Work out the finished part from the listing and answer in its coordinate system (mm). Face numbers are marked on the shaded views. A direction names the side the tool comes from. Coordinates: 2 decimals unless noted, no trailing zeros. Write each loop counter-clockwise with the first axis right and the second up, starting at its lowest first coordinate (ties: lowest second). Pieces come first, ordered by that corner, then holes. Notation, with made-up numbers: (28.5, 66) - (73.5, 66) arc R22 cw to (73.5, 77) - close; hole circle Ø1 at (11, 13). An arc over 180 degrees is marked (long way). Use a Markdown table: item, result. Add a question column.
(1) Find the intervals of material crossed by line 1 (X direction, y = 2.5, z = -1); line 2 (X direction, y = 5.5, z = -2); line 3 (X direction, y = 1.9, z = 6.75), in increasing order. Write a range as from..to.
(2) The part is cut by section B-B, the plane x = 20. Give the vertices of the cut face in (y, z).
(3) The part is cut by section C-C, the plane y = 1. Give the vertices of the cut face in (x, z).
(4) The part is cut by section A-A, the plane z = 0. Give the vertices of the cut face in (x, y), then the cut area to 4 significant figures.
(5) Given pin 1 Ø5.5 at (x, z) = (-20, 0) entering from -Y; pin 2 Ø2 at (x, y) = (5, 0.5) entering from +Z; pin 3 Ø2.5 at (x, y) = (4, 2) entering from -Z; pin 4 Ø3 at (x, y) = (-15.5, 1) entering from +Z, each flat-ended and moving along its own axis, determine where each tip first touches the part or whether it passes through.
(6) For a pull along X with two mould halves and no side action, classify the marked faces 4 and 5 as released by +X, released by -X, zero draft, split by the parting line, or undercut.
(7) A tool of negligible diameter and unlimited length cuts with its end or side. For the marked faces 1, 2 and 3, from which of +Z, -Z, +X, -X, +Y, -Y can it reach the whole face along a straight path? Write none if from no direction.
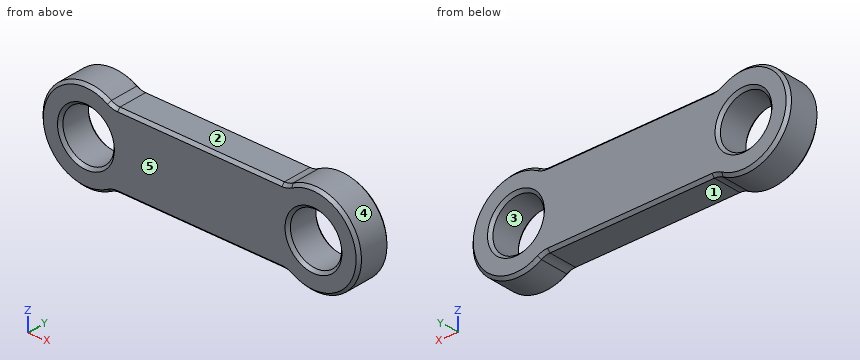
from build123d import *

# Parameters (mm, degrees)
SKETCH_1_R      = 4.5
EXTRUDE_1_DEPTH = 6
FILLET_1_R      = 3
CHAMFER_1_SIZE  = 0.5


with BuildPart() as part:
    # 草图1 → 凸台-拉伸1 (new body)
    with BuildSketch(Plane(origin=(0, 0, 0), x_dir=(1, 0, 0), z_dir=(0, 1, 0))):
        with BuildLine():
            Line((-15.336310473, 6.5), (15.336310473, 6.5))
            ThreePointArc((15.336310473, 6.5), (28, 0), (15.336310473, -6.5))
            Line((15.336310473, -6.5), (-15.336310473, -6.5))
            ThreePointArc((-15.336310473, -6.5), (-28, 0), (-15.336310473, 6.5))
        make_face()
        with Locations(Location((-20, 0, 0), (0, 0, 270))):
            Circle(SKETCH_1_R, mode=Mode.SUBTRACT)
        with Locations(Location((20, 0, 0), (0, 0, 270))):
            Circle(SKETCH_1_R, mode=Mode.SUBTRACT)
    extrude(amount=EXTRUDE_1_DEPTH)

    # 圆角1
    fillet_1_edges = [part.edges().sort_by_distance(p)[0] for p in [
        (-15.336310473, 3, -6.5),
        (15.336310473, 3, -6.5),
        (15.336310473, 3, 6.5),
        (-15.336310473, 3, 6.5),
    ]]
    fillet(fillet_1_edges, radius=FILLET_1_R)

    # 倒角1
    chamfer_1_edges = [part.edges().sort_by_distance(p)[0] for p in [
        (-20, 0, -4.5),
        (-20, 6, -4.5),
        (20, 0, -4.5),
        (20, 6, -4.5),
        (-28, 0, 0),
        (-28, 6, 0),
        (0, 0, -6.5),
        (0, 6, -6.5),
        (28, 0, 0),
        (28, 6, 0),
        (0, 0, 6.5),
        (0, 6, 6.5),
        (-15.238081199, 0, -6.604078103),
        (-15.238081199, 6, -6.604078103),
        (15.238081199, 0, -6.604078103),
        (15.238081199, 6, -6.604078103),
        (15.238081199, 0, 6.604078103),
        (15.238081199, 6, 6.604078103),
        (-15.238081199, 0, 6.604078103),
        (-15.238081199, 6, 6.604078103),
    ]]
    chamfer(chamfer_1_edges, length=CHAMFER_1_SIZE)


solid = part.part
Model answer:
| question | item | result |
|---|---|---|
| 1 | line 1 | -27.94..-24.39, -15.61..15.61, 24.39..27.94 |
| 1 | line 2 | -27.75..-24.03, -15.97..15.97, 24.03..27.75 |
| 1 | line 3 | -24.29..-15.65, 15.65..24.29 |
| 2 | outline | (0, -7.5) - (0.5, -8) - (5.5, -8) - (6, -7.5) - (6, -5) - (5.5, -4.5) - (0.5, -4.5) - (0, -5) - close; (0, 5) - (0.5, 4.5) - (5.5, 4.5) - (6, 5) - (6, 7.5) - (5.5, 8) - (0.5, 8) - (0, 7.5) - close |
| 3 | outline | (-15.97, -6.91) arc R3 cw to (-14.45, -6.5) - (14.45, -6.5) arc R3 cw to (15.97, -6.91) arc R8 ccw (long way) to (15.97, 6.91) arc R3 cw to (14.45, 6.5) - (-14.45, 6.5) arc R3 cw to (-15.97, 6.91) arc R8 ccw (long way) to start; hole circle Ø9 at (-20, 0); hole circle Ø9 at (20, 0) |
| 4 | outline | (-28, 0.5) - (-27.5, 0) - (-25, 0) - (-24.5, 0.5) - (-24.5, 5.5) - (-25, 6) - (-27.5, 6) - (-28, 5.5) - close; (-15.5, 0.5) - (-15, 0) - (15, 0) - (15.5, 0.5) - (15.5, 5.5) - (15, 6) - (-15, 6) - (-15.5, 5.5) - close; (24.5, 0.5) - (25, 0) - (27.5, 0) - (28, 0.5) - (28, 5.5) - (27.5, 6) - (25, 6) - (24.5, 5.5) - close |
| 4 | area | 226.5 mm^2 |
| 5 | pin 1 | through |
| 5 | pin 2 | z = 6.5 |
| 5 | pin 3 | z = -6.5 |
| 5 | pin 4 | z = 7.42 |
| 6 | face 4 | undercut |
| 6 | face 5 | zero draft |
| 7 | face 1 | -Z, +Y, -Y |
| 7 | face 2 | +Z, +Y, -Y |
| 7 | face 3 | +Y, -Y |
